from build123d import *

# Parameters (mm, degrees)
SKETCH_W        = 168
SKETCH_H        = 280
PAD_DEPTH       = 18
SKETCH001_W     = 168
SKETCH001_H     = 18
POCKET_DEPTH    = 9
SKETCH002_W     = 18
SKETCH002_H     = 280
POCKET001_DEPTH = 9
SKETCH003_W     = 168
SKETCH003_H     = 6
POCKET002_DEPTH = 6


with BuildPart() as part:
    # Sketch → Pad (new body)
    with BuildSketch(Plane.YZ):
        with Locations((-84, 140)):
            Rectangle(SKETCH_W, SKETCH_H)
    extrude(amount=PAD_DEPTH)

    # Sketch001 (on Face6 of Pad) → Pocket (cut)
    with BuildSketch(Plane.YZ.offset(18)):
        with Locations((-84, 9)):
            Rectangle(SKETCH001_W, SKETCH001_H)
        with Locations((-84, 177)):
            Rectangle(SKETCH001_W, SKETCH001_H)
        with Locations((-84, 261)):
            Rectangle(SKETCH001_W, SKETCH001_H)
    extrude(amount=-POCKET_DEPTH, mode=Mode.SUBTRACT)

    # Sketch002 (on Face35 of Pocket) → Pocket001 (cut)
    with BuildSketch(Plane.YZ.offset(18)):
        with Locations((-9, 140)):
            Rectangle(SKETCH002_W, SKETCH002_H)
    extrude(amount=-POCKET001_DEPTH, mode=Mode.SUBTRACT)

    # Sketch003 (on Face12 of Pocket001) → Pocket002 (cut)
    with BuildSketch(Plane.YZ.offset(18)):
        with Locations((-84, 21)):
            Rectangle(SKETCH003_W, SKETCH003_H)
        with Locations((-84, 96)):
            Rectangle(SKETCH003_W, SKETCH003_H)
    extrude(amount=-POCKET002_DEPTH, mode=Mode.SUBTRACT)


solid = part.part
Geometry: final body of the model. Coordinates: model frame, mm. A direction names the side the tool comes from. Give positions to 0.01 mm unless a question says otherwise; leave off trailing zeros. Write each loop counter-clockwise with the first axis right and the second up, starting at its lowest first coordinate (ties: lowest second). Pieces come first, ordered by that corner, then holes. Notation, with made-up numbers: M -25,60 L -2,60 A24 cw -2,93 Z; hole C 36.5,-23 d9. An arc over 180 degrees is marked long. Answer in a Markdown table with one row per item. Add a question column.
(1) Reachability of faces 1 (the flat face through (14, -18, 275)), 2 (the flat face through (14, -94, 252)), 3 (the flat face through (15, -94, 24)) from +Z, -Z, +X, -X, +Y, -Y: full face, straight path, thin tool, end or side. Return the list, or none.
(2) Section C-C on z = 182. Return loops of the section in (x, y), and give its area (3 significant figures).
(3) Section B-B on z = 112. Return loops of the section in (x, y), and give its area (3 significant figures).
(4) Mould query, pull axis Z, two halves, no side actions, for faces 4 (the flat face through (18, -94, 134)), 5 (the flat face through (4, -85, 0)), 6 (the flat face through (14, -94, 186)). Classes: +Z half, -Z half, draft (parallel to the pull), parting line (faces both ways), or undercut.
(5) First-contact query: pin 1 (2.5 mm diameter, centred on x = 12.5, z = 215, fed in from +Y); pin 2 (2.5 mm diameter, centred on x = 14.5, y = -96, fed in from -Z); pin 3 (3 mm diameter, centred on y = -56.5, z = 96, fed in from +X). Flat tips, straight axial feed; report the tip coordinate or a pass-through.
(6) Section A-A on y = -36.5. Return loops of the section in (x, z).
(7) Ray query, line 1 (Z direction, x = 9.25, y = -83); line 2 (Z direction, x = 14, y = -115.5); line 3 (X direction, y = -14, z = 106.5). Return the intervals inside material, ascending.
Result set:
| question | item | result |
|---|---|---|
| 1 | face 1 | +Z, -Z, +X, +Y |
| 1 | face 2 | +X, +Y, -Y |
| 1 | face 3 | -Z, +X, +Y, -Y |
| 2 | outline | M 0,-168 L 9,-168 L 9,0 L 0,0 Z |
| 2 | area | 1,510 mm^2 |
| 3 | outline | M 0,-168 L 18,-168 L 18,-18 L 9,-18 L 9,0 L 0,0 Z |
| 3 | area | 2,860 mm^2 |
| 4 | face 4 | draft |
| 4 | face 5 | -Z half |
| 4 | face 6 | undercut |
| 5 | pin 1 | stops at y = -18 |
| 5 | pin 2 | stops at z = 24 |
| 5 | pin 3 | stops at x = 12 |
| 6 | outline | M 0,0 L 9,0 L 9,18 L 12,18 L 12,24 L 18,24 L 18,93 L 12,93 L 12,99 L 18,99 L 18,168 L 9,168 L 9,186 L 18,186 L 18,252 L 9,252 L 9,270 L 18,270 L 18,280 L 0,280 Z |
| 7 | line 1 | z = 18 to 168, 186 to 252, 270 to 280 |
| 7 | line 2 | z = 24 to 93, 99 to 168, 186 to 252, 270 to 280 |
| 7 | line 3 | x = 0 to 9 |
